Input: part model. Units: mm. Frame: model coordinates. Face numbers are marked on the shaded views. A direction names the side the tool comes from. Round coordinates to 2 decimals unless told otherwise and drop trailing zeros. Write each loop counter-clockwise with the first axis right and the second up, starting at its lowest first coordinate (ties: lowest second). Pieces come first, ordered by that corner, then holes. Notation, with made-up numbers: M 68.25,73 L 84.25,73 A14 ccw 84.25,78 Z; hole C 27.25,11 d10. An arc over 180 degrees is marked long. Answer as CSV lines item,"result". Start each with the question number.
```python
from build123d import *

# Parameters (mm, degrees)
SKETCH087_W      = 12
SKETCH087_H      = 7
EXTRUDE007_DEPTH = 7
SKETCH088_W      = 2
SKETCH088_H      = 3
POCKET018_DEPTH  = 3.5
SKETCH089_R      = 0.75
HOLE018_DEPTH    = 12
HOLE018_TIPS_R   = 0.75


with BuildPart() as part:
    # Sketch087 → Extrude007 (new body)
    with BuildSketch(Plane.XY):
        with Locations((-134, -113.5)):
            Rectangle(SKETCH087_W, SKETCH087_H)
    extrude(amount=EXTRUDE007_DEPTH)

    # Sketch088 (on Face3 of Extrude007) → Pocket018 (cut)
    with BuildSketch(Plane.XZ.offset(117)):
        with Locations((-134, 3.5)):
            Rectangle(SKETCH088_W, SKETCH088_H)
    extrude(amount=-POCKET018_DEPTH, mode=Mode.SUBTRACT)

    # Sketch089 (on Face3 of Pocket018) → Hole018 (cut)
    with BuildSketch(Plane.YZ.offset(-128)):
        with Locations((-115.249997, 3.5)):
            Circle(SKETCH089_R)
    extrude(amount=-HOLE018_DEPTH, mode=Mode.SUBTRACT)

    # Hole018 tips → Hole018 tip 1 section 0
    with BuildSketch(Plane.YZ.offset(-140), mode=Mode.PRIVATE) as hole018_tip_1_s0:
        with Locations((-115.249997, 3.5)):
            Circle(HOLE018_TIPS_R)
    loft([hole018_tip_1_s0.sketch, Vertex(-140.450645, -115.249997, 3.5)], mode=Mode.SUBTRACT)


solid = part.part
```
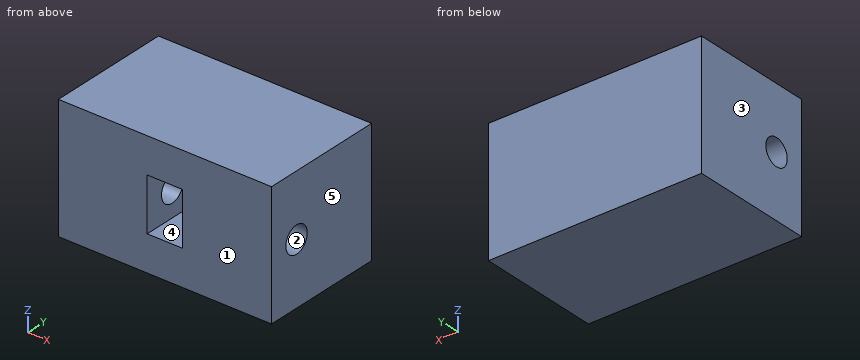
Item 1: Cut plane C-C, the plane x = -132.75. Return loops of the section in (y, z), plus the area to 3 significant figures.
Item 2: Line query: line 1 (X direction, y = -115, z = 2.5); line 2 (Z direction, x = -134.75, y = -114.5); line 3 (Y direction, x = -135.5, z = 3). Output: solid intervals per line, ascending. Write a range as [from, to].
Item 3: Pin query (flat end, axial travel): pin 1 Ø2 at (x, y) = (-134, -116) entering from -Z; pin 2 Ø1.6 at (x, z) = (-134, 4) entering from -Y. Return the tip coordinate at first contact, or that it passes through.
Item 4: Cut plane B-B, the plane z = 3.5. Return loops of the section in (x, y), plus the area to 3 significant figures.
Item 5: Draft query along Y for the marked faces 1, 2 and 3. Return one class per face: +Y half, -Y half, draft (parallel to the pull), parting line (faces both ways), or undercut.
Item 6: Access query for the marked faces 4 and 5. Directions: +Z, -Z, +X, -X, +Y, -Y. A direction counts if a zero-diameter tool reaches every point of the face in a straight line with its end or side. Return the directions, or none.
Item 7: Cut plane A-A, the plane y = -114. Return loops of the section in (x, z), plus the area to 3 significant figures.
Item 8: Cut plane D-D, the plane y = -115. Return loops of the section in (x, z).
Results list:
1,outline,"M -117,0 L -110,0 L -110,7 L -117,7 Z; hole C -115.25,3.5 d1.5"
1,area,"47.2 mm²"
2,line 1,"[-140, -135], [-133, -128]"
2,line 2,"[0, 2], [5, 7]"
2,line 3,"[-117, -115.81], [-114.69, -110]"
3,pin 1,"z = 0"
3,pin 2,"y = -113.5"
4,outline,"M -140,-117 L -135,-117 L -135,-116 L -140,-116 Z; M -140,-114.5 L -135,-114.5 L -135,-113.5 L -133,-113.5 L -133,-114.5 L -128,-114.5 L -128,-110 L -140,-110 Z; M -133,-117 L -128,-117 L -128,-116 L -133,-116 Z"
4,area,"62.0 mm²"
5,face 1,"-Y half"
5,face 2,"undercut"
5,face 3,"draft"
6,face 4,"-Y"
6,face 5,"+Z, -Z, +X, +Y, -Y"
7,outline,"M -140,0 L -128,0 L -128,7 L -140,7 Z; hole M -135,2 L -133,2 L -133,5 L -135,5 Z"
7,area,"78.0 mm²"
8,outline,"M -140,0 L -128,0 L -128,2.79 L -133,2.79 L -133,2 L -135,2 L -135,2.79 L -140,2.79 Z; M -140,4.21 L -135,4.21 L -135,5 L -133,5 L -133,4.21 L -128,4.21 L -128,7 L -140,7 Z"
